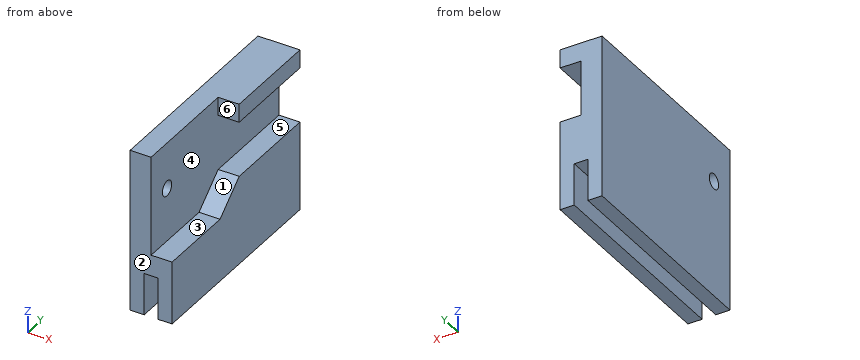
```python
from build123d import *

# Parameters (mm, degrees)
F1_DEPTH = 20
F3_DEPTH = 4
F4_R     = 1.45
F5_DEPTH = 25


with BuildPart() as f1:
    # F0 (on Front) → F1 (new body, symmetric)
    with BuildSketch(Plane.XZ):
        Polygon((4, -15.5), (4, 15.5), (-4, 15.5), (-4, -15.5), (-1.3, -15.5), (-1.3, -7.5), (1.3, -7.5), (1.3, -15.5), align=None)
    extrude(amount=F1_DEPTH, both=True)

    # F2 (on face) → F3 (cut, through all)
    with BuildSketch(Plane.YZ.offset(4)):
        Polygon((-20, 15.5), (-20, -3.5), (-5, -3.5), (1, 1.5), (20, 1.5), (20, 12), (1, 12), (1, 15.5), align=None)
    extrude(amount=-F3_DEPTH, mode=Mode.SUBTRACT)

    # F4 (on face) → F5 (cut)
    with BuildSketch(Plane.YZ):
        with Locations((-15, 6.7)):
            Circle(F4_R)
    extrude(amount=-F5_DEPTH, mode=Mode.SUBTRACT)


solid = f1.part
```
Check sheet for the modelled part. Datum: model origin and axes. Units: mm. Face numbers are marked on the shaded views. A direction names the side the tool comes from. Round coordinates to 2 decimals unless told otherwise and drop trailing zeros. Loops run counter-clockwise (first coordinate to the right, second up) from the corner with the lowest first, then second, coordinate; pieces in that order, holes last. Notation, with made-up numbers: (37.5, 80) - (58.5, 80) arc R21 cw to (58.5, 92) - close; hole circle Ø3 at (43.25, -27.5). An arc over 180 degrees is marked (long way). Answer as a JSON object with one key per item and string values. Group by question number.
Q1. Set-up check for the marked faces 1 and 2: record each of +Z, -Z, +X, -X, +Y, -Y from which the full face is reachable in a straight line by a thin tool's end or side.
Q2. Gauge pin test, flat ends, axial feed: P1, Ø1, axis at x = 3, y = -0.5, coming from the +Z side; P2, Ø1.3, axis at x = 0.5, y = -6, coming from the -Z side; P3, Ø2.5, axis at y = -15, z = 6.7, coming from the +X side; P4, Ø1.2, axis at x = 2.5, y = -12.5, coming from the +Z side. Record the tip position at first contact, or that the pin passes through.
Q3. Mould release check, pull along Z, two halves, no side actions. Record for the marked faces 3, 4, 5 and 6: released by +Z, released by -Z, zero draft, split by the parting line, or undercut.
Q4. Sectioned sample at A-A, the plane x = 0.5. Enter the section's corners in (y, z).
Q5. Sectioned sample at D-D, the plane y = -11. Enter the section's corners in (x, z).
Q6. Sectioned sample at B-B, the plane z = 6.7. Enter the section's corners in (x, y), plus the area to 3 significant figures.
Q7. Scan lines: line 1 along Z through (x, y) = (-2.75, -15); line 2 along X through (y, z) = (9.5, -13); line 3 along Z through (x, y) = (-1.1, -15). Record each from-to range of solid material in increasing order. Write a range as [from, to].
Q8. Sectioned sample at C-C, the plane y = -15. Enter the section's corners in (x, z).
Solution:
{
 "1": {"face 1": "+Z, +X, -Y", "face 2": "+Z, -Z, +X, -X, -Y"},
 "2": {"P1": "stops at z = 0.67", "P2": "stops at z = -7.5", "P3": "passes through", "P4": "stops at z = -3.5"},
 "3": {"face 3": "released by +Z", "face 4": "undercut", "face 5": "undercut", "face 6": "zero draft"},
 "4": {"outline": "(-20, -7.5) - (20, -7.5) - (20, 1.5) - (1, 1.5) - (-5, -3.5) - (-20, -3.5) - close; (1, 12) - (20, 12) - (20, 15.5) - (1, 15.5) - close"},
 "5": {"outline": "(-4, -15.5) - (-1.3, -15.5) - (-1.3, -7.5) - (1.3, -7.5) - (1.3, -15.5) - (4, -15.5) - (4, -3.5) - (0, -3.5) - (0, 15.5) - (-4, 15.5) - close"},
 "6": {"outline": "(-4, -20) - (0, -20) - (0, -16.45) - (-4, -16.45) - close; (-4, -13.55) - (0, -13.55) - (0, 20) - (-4, 20) - close", "area": "148 mm²"},
 "7": {"line 1": "z = [-15.5, 5.25], [8.15, 15.5]", "line 2": "x = [-4, -1.3], [1.3, 4]", "line 3": "z = [-7.5, 5.25], [8.15, 15.5]"},
 "8": {"outline": "(-4, -15.5) - (-1.3, -15.5) - (-1.3, -7.5) - (1.3, -7.5) - (1.3, -15.5) - (4, -15.5) - (4, -3.5) - (0, -3.5) - (0, 5.25) - (-4, 5.25) - close; (-4, 8.15) - (0, 8.15) - (0, 15.5) - (-4, 15.5) - close"}
}
